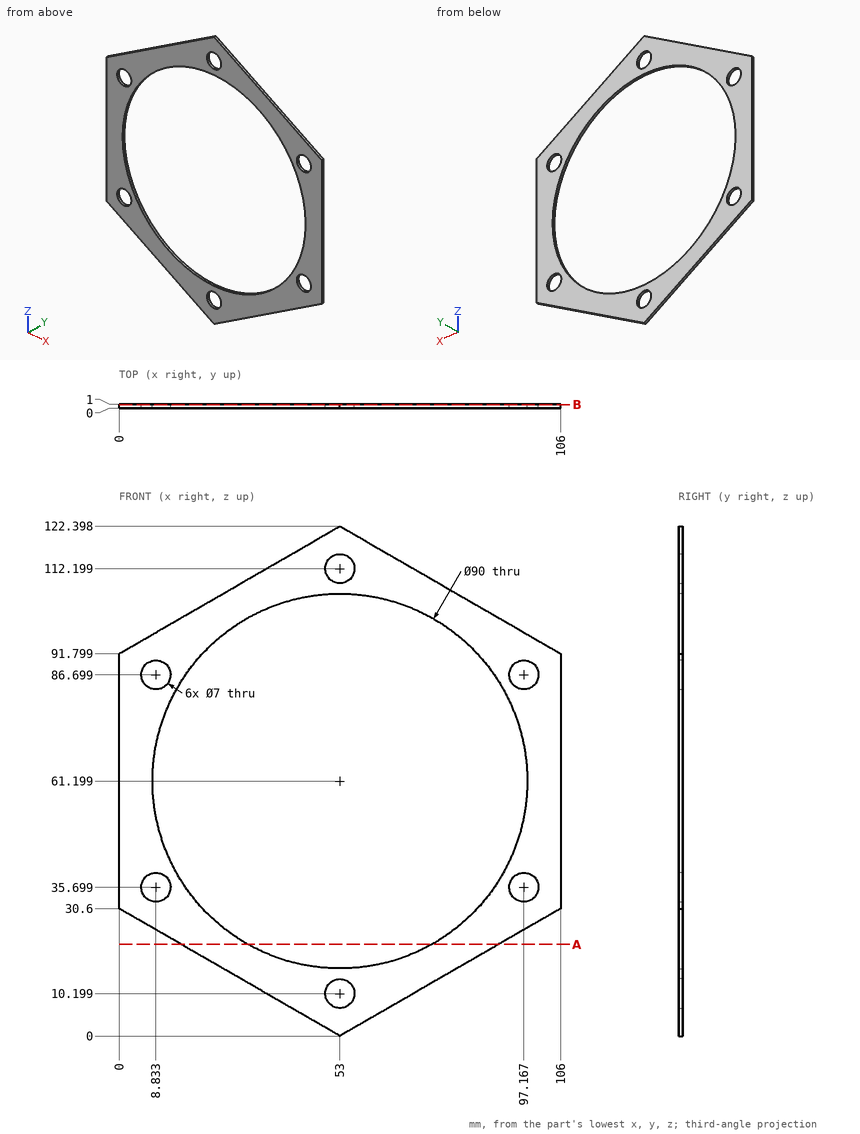
Print and shaded views of the part. All mm, measured from the part's lowest x, y and z. Round coordinates to 2 decimals unless told otherwise and drop trailing zeros. Write each loop counter-clockwise with the first axis right and the second up, starting at its lowest first coordinate (ties: lowest second). Pieces come first, ordered by that corner, then holes.
Item 1: Cut at A-A, the plane z = 22. Give the cut face in (x, y) (1 decimal).
Results:
outline: (14.9, 0) - (30.9, 0) - (30.9, 1) - (14.9, 1) - close; (75.1, 0) - (91.1, 0) - (91.1, 1) - (75.1, 1) - close
Item 2: Drop a flat-ended pin along its axis: pin 1 Ø9 at (x, z) = (97.17, 35.7) entering from +Y. Give the stop position or say it passes through.
Results:
pin 1: stops at y = 1
Item 3: Cut at B-B, the plane y = 0.85. Give the cut face in (x, z).
Results:
outline: (0, 30.6) - (53, 0) - (106, 30.6) - (106, 91.8) - (53, 122.4) - (0, 91.8) - close; hole circle Ø7 at (8.83, 35.7); hole circle Ø7 at (8.83, 86.7); hole circle Ø90 at (53, 61.2); hole circle Ø7 at (53, 10.2); hole circle Ø7 at (53, 112.2); hole circle Ø7 at (97.17, 35.7); hole circle Ø7 at (97.17, 86.7)
Item 4: Probe L1, parallel to X at y = 0.45, z = 36.5 (1 decimal); L2, parallel to Z at x = 19, y = 0.2; L3, parallel to X at y = 0.95, z = 29.5 (1 decimal). List the from-to ranges inside material, lowest first.
Results:
L1: x = 0 to 5.4, 12.2 to 15.4, 90.6 to 93.8, 100.6 to 106
L2: z = 19.63 to 31.72, 90.68 to 102.77
L3: x = 1.9 to 21.1, 84.9 to 104.1
